Geometry check sheet. Reference: the model listing, model coordinates, mm. Face numbers are marked on the shaded views. A direction names the side the tool comes from. Coordinates: 2 decimals unless noted, no trailing zeros. Write each loop counter-clockwise with the first axis right and the second up, starting at its lowest first coordinate (ties: lowest second). Pieces come first, ordered by that corner, then holes. Notation, with made-up numbers: (53, 36) -> (68, 36) arc R13 ccw to (68, 43) -> close; hole circle Ø10 at (61, 86). An arc over 180 degrees is marked (long way). Answer in a Markdown table with one row per item. Add a question column.
Q1. Section check A-A, the plane y = 2.5. Record the boundary of the cut face in (x, z), and give its area (3 significant figures).
Q2. Section check C-C, the plane x = -4.5. Record the boundary of the cut face in (y, z), and give its area (3 significant figures).
Q3. Release check for a two-part mould opening along X. For the marked faces 4, 5 and 6 record: pulls with the +X half, pulls with the -X half, needs draft (parallel to the pull), parting line crosses it, or undercut.
Q4. Section check B-B, the plane x = 1. Record the boundary of the cut face in (y, z), and give its area (3 significant figures).
Q5. Tool access check on the marked faces 1, 2 and 3. Record the directions out of +Z, -Z, +X, -X, +Y, -Y that give a thin tool (end or side, any length) a straight path to the whole face; none if there is none.
Q6. Gauge pin test, flat ends, axial feed: P1, Ø2, axis at x = 3, z = -0.5, coming from the -Y side; P2, Ø6, axis at x = -1.5, y = -1, coming from the +Z side; P3, Ø0.6, axis at x = 0, y = -12.5, coming from the -Z side; P4, Ø1, axis at y = -4, z = 1, coming from the +X side. Record the tip position at first contact, or that the pin passes through.
Q7. Thickness scan on line 1 (Y direction, x = -3.25, z = -0.7); line 2 (X direction, y = -11.5, z = -1.6); line 3 (Z direction, x = 3, y = -2). Record the ranges inside material, lowest first.
```python
from build123d import *

# Parameters (mm, degrees)
F0_W     = 11
F0_H     = 20
F1_DEPTH = 2.5
F2_W     = 8
F2_H     = 17
F3_DEPTH = 1.2
F4_R     = 0.4
F5_R     = 0.6
F6_W     = 1.1
F6_H     = 6.5
F7_DEPTH = 2
F8_R     = 2
F9_DEPTH = 25
F10_R    = 1


with BuildPart() as f1:
    # F0 (on Top) → F1 (new body)
    with BuildSketch(Plane.XY):
        Rectangle(F0_W, F0_H)
    extrude(amount=-F1_DEPTH)

    # F2 (on face) → F3 (cut)
    with BuildSketch(Plane.XY):
        Rectangle(F2_W, F2_H)
    extrude(amount=-F3_DEPTH, mode=Mode.SUBTRACT)

    # F4
    f4_edges = [f1.edges().sort_by_distance(p)[0] for p in [
        (4, 0, -1.2),
        (0, 8.5, -1.2),
        (-4, 0, -1.2),
        (0, -8.5, -1.2),
    ]]
    fillet(f4_edges, radius=F4_R)

    # F5
    f5_edges = [f1.edges().sort_by_distance(p)[0] for p in [
        (5.5, 0, -2.5),
        (0, 10, -2.5),
        (-5.5, 0, -2.5),
        (0, -10, -2.5),
        (5.5, -10, -1.25),
        (-5.5, -10, -1.25),
        (-5.5, 10, -1.25),
        (5.5, 10, -1.25),
    ]]
    fillet(f5_edges, radius=F5_R)

    # F6 (on face) → F7 (join, symmetric)
    with BuildSketch(Plane.XY):
        with Locations((0, -13)):
            Rectangle(F6_W, F6_H)
    extrude(amount=F7_DEPTH, both=True)

    # F8 (on face) → F9 (cut)
    with BuildSketch(Plane.YZ.offset(0.55)):
        with Locations((-9.75, 2)):
            Circle(F8_R)
    extrude(amount=-F9_DEPTH, mode=Mode.SUBTRACT)

    # F10
    f10_edges = [f1.edges().sort_by_distance(p)[0] for p in [
        (0, -16.25, 2),
        (0, -16.25, -2),
        (0, -11.75, 2),
    ]]
    fillet(f10_edges, radius=F10_R)


solid = f1.part
```
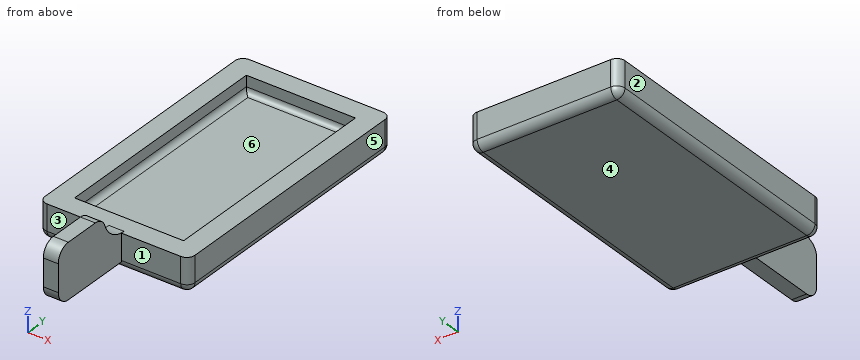
Calculated:
| question | item | result |
|---|---|---|
| 1 | outline | (-5.5, -1.9) arc R0.6 ccw to (-4.9, -2.5) -> (4.9, -2.5) arc R0.6 ccw to (5.5, -1.9) -> (5.5, 0) -> (4, 0) -> (4, -0.8) arc R0.4 cw to (3.6, -1.2) -> (-3.6, -1.2) arc R0.4 cw to (-4, -0.8) -> (-4, 0) -> (-5.5, 0) -> close |
| 1 | area | 17.8 mm² |
| 2 | outline | (-10, -1.9) arc R0.6 ccw to (-9.4, -2.5) -> (9.4, -2.5) arc R0.6 ccw to (10, -1.9) -> (10, 0) -> (-10, 0) -> close |
| 2 | area | 49.8 mm² |
| 3 | face 4 | needs draft |
| 3 | face 5 | pulls with the +X half |
| 3 | face 6 | undercut |
| 4 | outline | (-10, -1.9) arc R0.6 ccw to (-9.4, -2.5) -> (9.4, -2.5) arc R0.6 ccw to (10, -1.9) -> (10, 0) -> (8.5, 0) -> (8.5, -0.8) arc R0.4 cw to (8.1, -1.2) -> (-8.1, -1.2) arc R0.4 cw to (-8.5, -0.8) -> (-8.5, 0) -> (-10, 0) -> close |
| 4 | area | 29.5 mm² |
| 5 | face 1 | +Z, -Z, +X, -Y |
| 5 | face 2 | +Z, -Z, -X, +Y, -Y |
| 5 | face 3 | +Z, -Z, -X, -Y |
| 6 | P1 | stops at y = -10 |
| 6 | P2 | stops at z = 0 |
| 6 | P3 | stops at z = -2 |
| 6 | P4 | passes through |
| 7 | line 1 | y = -10 to -8.5, 8.5 to 10 |
| 7 | line 2 | x = -0.55 to 0.55 |
| 7 | line 3 | z = -2.5 to -1.2 |
